Read the model definition and answer for the solid it produces. Units are mm, in the model's axes. A direction names the side the tool comes from. Coordinates: 2 decimals unless noted, no trailing zeros. Write each loop counter-clockwise with the first axis right and the second up, starting at its lowest first coordinate (ties: lowest second). Pieces come first, ordered by that corner, then holes. Notation, with made-up numbers: (12.25, -14.75) -> (66.25, -14.75) arc R26 cw to (66.25, 11.25) -> close; hole circle Ø6 at (-16, 0.25). An arc over 180 degrees is marked (long way). Return JSON: item names as keys, results as strings.
from build123d import *

# Parameters (mm, degrees)
PAD_DEPTH       = 3
PAD001_DEPTH    = 3
SKETCH002_W     = 209.08447
SKETCH002_H     = 4.18
PAD002_DEPTH    = 3
SKETCH003_W     = 26.3
SKETCH003_H     = 34.2
POCKET_DEPTH    = 3
SKETCH004_W     = 18
SKETCH004_H     = 25
POCKET001_DEPTH = 3
SKETCH005_W     = 14
SKETCH005_H     = 5
POCKET002_DEPTH = 6
SKETCH006_W     = 14
SKETCH006_H     = 3
POCKET003_DEPTH = 3


with BuildPart() as part:
    # Sketch → Pad (new body)
    with BuildSketch(Plane.XY):
        with BuildLine():
            ThreePointArc((-100, 50), (-150, 0), (-100, -50))
            Line((-100, -50), (100, -50))
            ThreePointArc((100, -50), (150, 0), (100, 50))
            Line((-100, 50), (100, 50))
        make_face()
    extrude(amount=PAD_DEPTH)

    # Sketch001 (on Face6 of Pad) → Pad001 (join)
    with BuildSketch(Plane.XY.offset(3)):
        with BuildLine():
            ThreePointArc((-100, 50), (-150, 0), (-100, -50))
            Line((-100, -50), (100, -50))
            ThreePointArc((100, -50), (150, 0), (100, 50))
            Line((-100, 50), (100, 50))
        make_face()
        with BuildLine():
            ThreePointArc((-100, 5), (-105, 0), (-100, -5))
            Line((-100, -5), (100, -5))
            ThreePointArc((100, -5), (105, 0), (100, 5))
            Line((-100, 5), (100, 5))
        make_face(mode=Mode.SUBTRACT)
    extrude(amount=PAD001_DEPTH)

    # Sketch002 (on Face9 of Pad001) → Pad002 (join)
    with BuildSketch(Plane.XY.offset(6)):
        with BuildLine():
            ThreePointArc((-100, 50), (-150, 0), (-100, -50))
            Line((-100, -50), (100, -50))
            ThreePointArc((100, -50), (150, 0), (100, 50))
            Line((-100, 50), (100, 50))
        make_face()
        Rectangle(SKETCH002_W, SKETCH002_H, mode=Mode.SUBTRACT)
    extrude(amount=PAD002_DEPTH)

    # Sketch003 (on Face13 of Pad002) → Pocket (cut)
    with BuildSketch(Plane.XY.offset(9)):
        with Locations((0, -29.9)):
            Rectangle(SKETCH003_W, SKETCH003_H)
    extrude(amount=-POCKET_DEPTH, mode=Mode.SUBTRACT)

    # Sketch004 (on Face27 of Pocket) → Pocket001 (cut)
    with BuildSketch(Plane.XY.offset(6)):
        with Locations((0, -25.3)):
            Rectangle(SKETCH004_W, SKETCH004_H)
    extrude(amount=-POCKET001_DEPTH, mode=Mode.SUBTRACT)

    # Sketch005 (on Face13 of Pocket001) → Pocket002 (cut)
    with BuildSketch(Plane.XY.offset(9)):
        with Locations((0, -10.3)):
            Rectangle(SKETCH005_W, SKETCH005_H)
    extrude(amount=-POCKET002_DEPTH, mode=Mode.SUBTRACT)

    # Sketch006 (on Face23 of Pocket002) → Pocket003 (cut)
    with BuildSketch(Plane.XZ.offset(7.8)):
        with Locations((0, 4.5)):
            Rectangle(SKETCH006_W, SKETCH006_H)
    extrude(amount=-POCKET003_DEPTH, mode=Mode.SUBTRACT)


solid = part.part
1. Consider L1, parallel to Y at x = -60.5, z = 3.5; L2, parallel to Y at x = 0, z = 4; L3, parallel to X at y = -4, z = 5. Determine where each line is inside the solid, lowest interval first.
Taken from the geometry:
{"L1": "y = -50 to -5, 5 to 50", "L2": "y = -50 to -37.8, 5 to 50", "L3": "x = -149.84 to -103, 103 to 149.84"}
2. For a pull along X with two mould halves and no side action, classify faces 4 (the face through (-1, 50, 4)), 5 (the face through (149.988, -1.099, 4.437)), 6 (the face through (7, -10, 6)), 7 (the face through (-1, -4, 6)) as +X half, -X half, draft (parallel to the pull), parting line (faces both ways), or undercut.
Taken from the geometry:
{"face 4": "draft", "face 5": "+X half", "face 6": "undercut", "face 7": "undercut"}
3. A tool of negligible diameter and unlimited length cuts with its end or side. For faces 1 (the face through (-149.988, 1.099, 4.437)), 2 (the face through (105, 0, 4)), 3 (the face through (9, -12.8, 7)), from which of +Z, -Z, +X, -X, +Y, -Y can it reach the whole face along a straight path? Write none if from no direction.
Taken from the geometry:
{"face 1": "+Z, -Z, -X", "face 2": "none", "face 3": "+Z"}
4. The part is cut by section B-B (y = -24.5). Determine the outline of the cut face in (x, z), then the cut area to 3 significant figures.
Taken from the geometry:
{"outline": "(-143.59, 0) -> (143.59, 0) -> (143.59, 9) -> (13.15, 9) -> (13.15, 6) -> (9, 6) -> (9, 3) -> (-9, 3) -> (-9, 6) -> (-13.15, 6) -> (-13.15, 9) -> (-143.59, 9) -> close", "area": "2,450 mm2"}
5. Flat-ended cylindrical pins translate along their axes: pin 1 Ø2 at (y, z) = (32, 4) entering from +X; pin 2 Ø0.9 at (y, z) = (-23.5, 7.5) entering from +X; pin 3 Ø2.5 at (y, z) = (1, 8) entering from -X. Find the tip coordinate at first contact, or state that the pin passes through.
Taken from the geometry:
{"pin 1": "stops at x = 139.23", "pin 2": "stops at x = 144.37", "pin 3": "stops at x = -150"}
6. The part is cut by section A-A (x = -57.5). Determine the outline of the cut face in (y, z).
Taken from the geometry:
{"outline": "(-50, 0) -> (50, 0) -> (50, 9) -> (2.09, 9) -> (2.09, 6) -> (5, 6) -> (5, 3) -> (-5, 3) -> (-5, 6) -> (-2.09, 6) -> (-2.09, 9) -> (-50, 9) -> close"}
7. The part is cut by section C-C (x = 131.5). Determine the outline of the cut face in (y, z).
Taken from the geometry:
{"outline": "(-38.83, 0) -> (38.83, 0) -> (38.83, 9) -> (-38.83, 9) -> close"}
